Geometry check sheet. Reference: the model listing, model coordinates, mm. A direction names the side the tool comes from. Coordinates: 2 decimals unless noted, no trailing zeros. Write each loop counter-clockwise with the first axis right and the second up, starting at its lowest first coordinate (ties: lowest second). Pieces come first, ordered by that corner, then holes. Notation, with made-up numbers: (40.5, 20) -> (99.5, 20) arc R21 ccw to (99.5, 45) -> close; hole circle Ø9 at (82.25, -8.5). An arc over 180 degrees is marked (long way). Answer in a Markdown table with one row per item. Add a question column.
Q1. Tool access check on faces 1 (the face through (25, 130, -9)), 2 (the face through (10.05, 24.65, -228.38)). Record the directions out of +Z, -Z, +X, -X, +Y, -Y that give a thin tool (end or side, any length) a straight path to the whole face; none if there is none.
Q2. Thickness scan on line 1 (X direction, y = 17, z = 0) (3 decimals); line 2 (Z direction, x = 128, y = 29); line 3 (Z direction, x = -6, y = 91.5). Record the ranges inside material, lowest first.
Q3. Gauge pin test, flat ends, axial feed: P1, Ø6, axis at x = -102.5, y = 91.5, coming from the +Z side; P2, Ø2, axis at y = 82.5, z = 162, coming from the +X side; P3, Ø4, axis at x = 29, z = -106, coming from the +Y side. Record the tip position at first contact, or that the pin passes through.
Q4. Section check A-A, the plane y = 15. Record the boundary of the cut face in (x, z) (3 decimals), and give its area (3 significant figures).
Q5. Release check for a two-part mould opening along X. For faces 3 (the face through (29.893, 169.849, -3.925)), 4 (the face through (29.893, 134.86, -3.925)), 5 (the face through (217.21, 24.65, -28.52)), 6 (the face through (-117.5, 0, 185.2)) record: pulls with the +X half, pulls with the -X half, needs draft (parallel to the pull), parting line crosses it, or undercut.
Q6. Section check B-B, the plane y = 165. Record the boundary of the cut face in (x, z), and give its area (3 significant figures).
```python
from build123d import *

# Parameters (mm, degrees)
CROQUIS1_R              = 228.6
SALIENTE_EXTRUIR1_DEPTH = 50
C_PULA1_FACE_RADIUS     = 228.6
C_PULA1_HEIGHT          = 100
VACIADO1_T              = -9.525
CROQUIS3_R              = 30.15
SALIENTE_EXTRUIR2_DEPTH = 60
CORTAR_EXTRUIR1_REACH   = 376.988
CROQUIS4_R              = 26.24


with BuildPart() as part:
    # Croquis1 → Saliente-Extruir1 (new body)
    with BuildSketch(Plane(origin=(0, 0, 0), x_dir=(1, 0, 0), z_dir=(0, 1, 0))):
        with Locations(Location((0, 0, 0), (0, 0, 270))):
            Circle(CROQUIS1_R)
    extrude(amount=SALIENTE_EXTRUIR1_DEPTH)

    # C_pula1: an elliptical dome of height H over a round flat face of radius A is half a spheroid: the quarter ellipse of half axes A and H revolved about the face's axis
    with BuildSketch(Plane((0, 50, 0), x_dir=(0, 0, -1), z_dir=(1, 0, 0)), mode=Mode.PRIVATE) as c_pula1_quarter:
        Ellipse(C_PULA1_FACE_RADIUS, C_PULA1_HEIGHT)
        Rectangle(C_PULA1_FACE_RADIUS, C_PULA1_HEIGHT, align=(Align.MIN, Align.MIN), mode=Mode.INTERSECT)
    revolve(c_pula1_quarter.sketch, axis=Axis((0, 50, 0), (0, 1, 0)))

    # Vaciado1
    vaciado1_openings = [part.faces().sort_by_distance(p)[0] for p in [
        (0, 0, 0),
    ]]
    offset(amount=VACIADO1_T, openings=vaciado1_openings, kind=Kind.INTERSECTION)

    # Croquis3 → Saliente-Extruir2 (add)
    with BuildSketch(Plane(origin=(0, 190, 0), x_dir=(1, 0, 0), z_dir=(0, 1, 0))):
        with Locations(Location((0, 0, 0), (0, 0, 270))):
            Circle(CROQUIS3_R)
    extrude(amount=-SALIENTE_EXTRUIR2_DEPTH)

    # Croquis4 → Cortar-Extruir1 (cut, up to next)
    with BuildSketch(Plane(origin=(0, 190, 0), x_dir=(1, 0, 0), z_dir=(0, 1, 0)), mode=Mode.PRIVATE) as cortar_extruir1_sk1:
        with Locations(Location((0, 0, 0), (0, 0, 270))):
            Circle(CROQUIS4_R)
    cortar_extruir1_tool1 = extrude(cortar_extruir1_sk1.sketch, amount=-CORTAR_EXTRUIR1_REACH, mode=Mode.PRIVATE) & part.part
    add(cortar_extruir1_tool1.solids().sort_by_distance((0, 190, 0))[0], mode=Mode.SUBTRACT)


solid = part.part
```
Calculated:
| question | item | result |
|---|---|---|
| 1 | face 1 | -Y |
| 1 | face 2 | +Y, -Y |
| 2 | line 1 | x = -228.6 to -219.075, 219.075 to 228.6 |
| 2 | line 2 | z = -189.4 to -177.79, 177.79 to 189.4 |
| 2 | line 3 | z = -207.9 to -193.31, 193.31 to 207.9 |
| 3 | P1 | stops at z = 184.8 |
| 3 | P2 | stops at x = 144.78 |
| 3 | P3 | stops at y = 138.16 |
| 4 | outline | circle Ø457.2 at (0, 0); hole circle Ø438.15 at (0, 0) |
| 4 | area | 13,400 mm² |
| 5 | face 3 | parting line crosses it |
| 5 | face 4 | undercut |
| 5 | face 5 | undercut |
| 5 | face 6 | needs draft |
| 6 | outline | circle Ø60.3 at (0, 0); hole circle Ø52.48 at (0, 0) |
| 6 | area | 693 mm² |
